Check sheet for the drawn part. Datum: minimum x, y, z corner. Units: mm. A direction names the side the tool comes from. Coordinates: 2 decimals unless noted, no trailing zeros. Order: outer loops, then holes, each group sorted by start corner. A loop starts at its lowest first (then second) coordinate and runs counter-clockwise, first axis right, second up.
Q1. Draft check along Y on the marked faces 4, 5 and 6. Enter one of: pulls with the +Y half, pulls with the -Y half, needs draft (parallel to the pull), parting line crosses it, or undercut.
Q2. Cross-section at D-D, the plane x = 27.5. Record the boundary of the cut face in (y, z).
Q3. Depth check by flat-ended pin: P1, Ø2.5, axis at y = 27.5, z = 31.5, coming from the -X side (1 decimal); P2, Ø4, axis at y = 19, z = 1.5, coming from the +X side (1 decimal); P3, Ø8, axis at x = 29, z = 25.5, coming from the -Y side. Enter the tip coordinate at first touch or a pass-through.
Q4. Thickness scan on line 1 (Z direction, x = 20, y = 12); line 2 (Y direction, x = 38, z = 10.5); line 3 (Y direction, x = 12, z = 32). Record the ranges inside material, lowest first.
Q5. Cross-section at A-A, the plane y = 12.5. Record the boundary of the cut face in (x, z), and give its area (3 significant figures).
Q6. Set-up check for the marked faces 1, 2 and 3: record each of +Z, -Z, +X, -X, +Y, -Y from which the full face is reachable in a straight line by a thin tool's end or side.
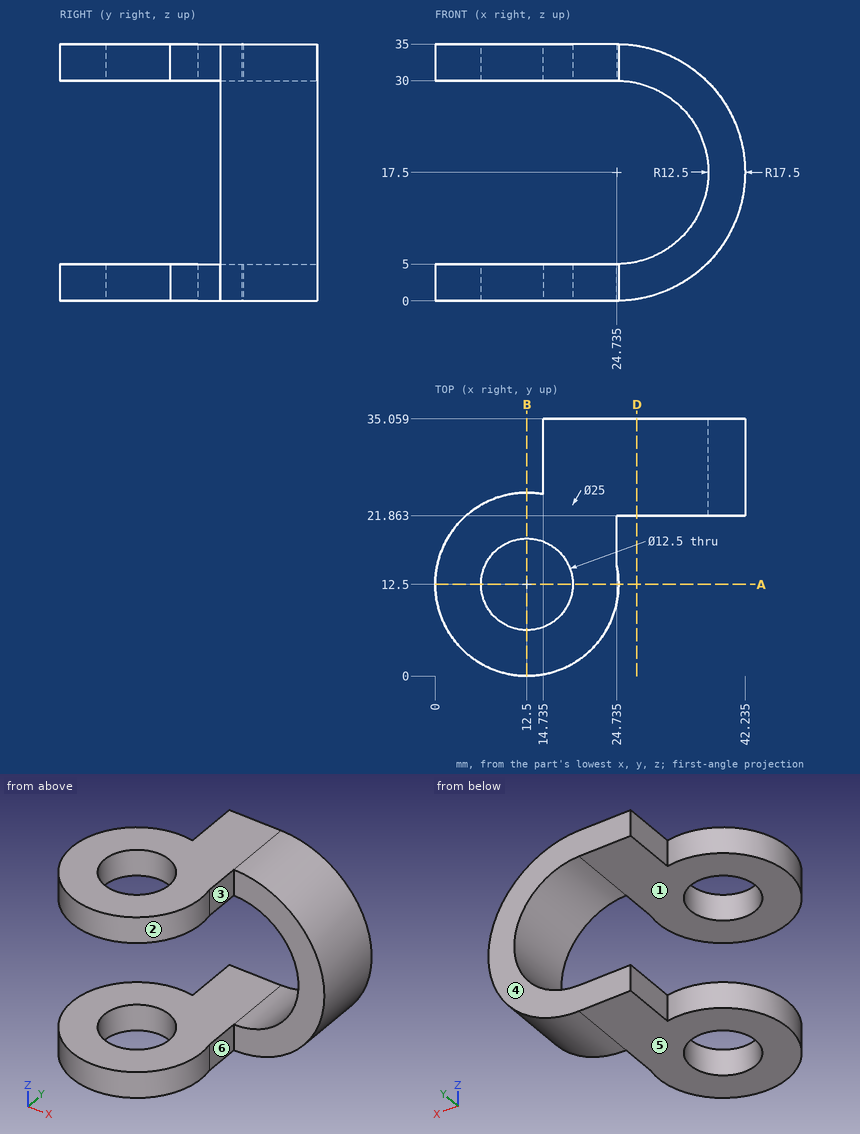
Check values:
1. face 4: pulls with the +Y half
1. face 5: needs draft
1. face 6: undercut
2. outline: (21.86, 0.22) - (35.06, 0.22) - (35.06, 5.31) - (21.86, 5.31) - close; (21.86, 29.69) - (35.06, 29.69) - (35.06, 34.78) - (21.86, 34.78) - close
3. P1: stops at x = 14.7
3. P2: stops at x = 24.7
3. P3: stops at y = 21.86
4. line 1: z = 0 to 5, 30 to 35
4. line 2: y = 21.86 to 35.06
4. line 3: y = 0.01 to 6.27, 18.73 to 24.99
5. outline: (0, 0) - (6.25, 0) - (6.25, 5) - (0, 5) - close; (0, 30) - (6.25, 30) - (6.25, 35) - (0, 35) - close; (18.75, 0) - (25, 0) - (25, 5) - (18.75, 5) - close; (18.75, 30) - (25, 30) - (25, 35) - (18.75, 35) - close
5. area: 125 mm2
6. face 1: -X, +Y, -Y
6. face 2: +Z, -Z
6. face 3: +Z, -Z, +X
